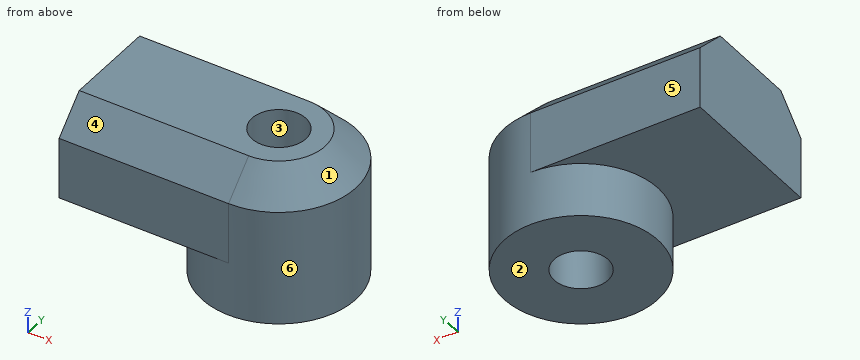
from build123d import *

# Parameters (mm, degrees)
F1_DEPTH = 6
F2_R     = 5
F2_R_2   = 1.75
F3_DEPTH = 9.5
F4_SIZE  = 2


with BuildPart() as f1:
    # F0 (on Top) → F1 (new body)
    with BuildSketch(Plane.XY):
        with BuildLine():
            ThreePointArc((0, -5), (-5, 0), (0, 5))
            Line((0, 5), (-11, 5))
            Line((-11, 5), (-11, -5))
            Line((-11, -5), (0, -5))
        make_face()
    extrude(amount=-F1_DEPTH)

    # F2 (on Top) → F3 (join)
    with BuildSketch(Plane.XY):
        Circle(F2_R)
        Circle(F2_R_2, mode=Mode.SUBTRACT)
    extrude(amount=-F3_DEPTH)

    # F4
    f4_edges = [f1.edges().sort_by_distance(p)[0] for p in [
        (-5.5, 5, 0),
    ]]
    chamfer(f4_edges, length=F4_SIZE)


solid = f1.part
Design review of the part built by this model. Coordinates are the model's own, in mm. Face numbers are marked on the shaded views. A direction names the side the tool comes from. Round coordinates to 2 decimals unless told otherwise and drop trailing zeros. Write each loop counter-clockwise with the first axis right and the second up, starting at its lowest first coordinate (ties: lowest second). Pieces come first, ordered by that corner, then holes. Notation, with made-up numbers: M -0.5,-36.75 L 47.5,-36.75 A32 ccw 47.5,-7.75 Z; hole C -34,-10 d10. An arc over 180 degrees is marked long. One line per item, written item: value. Start each with the question number.
1. Clearance check with flat-ended pins moving along their axes: P1, Ø1.5, axis at y = -1.5, z = -8, coming from the +X side; P2, Ø2, axis at y = -3, z = -7.5, coming from the +X side. State where each tip first meets the part, or that it passes through.
2. Draft analysis for pull direction Y (two halves, no side actions). For the marked faces 1, 2, 3 and 4, state which applies: pulls with the +Y half, pulls with the -Y half, needs draft (parallel to the pull), parting line crosses it, or undercut.
3. Take a section at D-D on z = -5. State the section outline as (x, y) points, then the cut area to 3 significant figures.
4. To check wall thickness, follow probe 1 along Z at (x, y) = (-9.5, -0.5); probe 2 along X at (y, z) = (0.25, -5.5); probe 3 along X at (y, z) = (-1.5, -6.75). State the ranges of each line that lie inside material, in increasing order. Write a range as from..to.
5. For the marked faces 5 and 6, list the 3-axis set-ups (+Z, -Z, +X, -X, +Y, -Y) from which the entire face can be reached by the end or side of a thin tool; tool diameter is ignored.
6. Take a section at C-C on x = -6.75. State the section outline as (y, z) points.
7. Take a section at A-A on y = 0. State the section outline as (x, z) points, then the cut area to 4 significant figures.
8. Take a section at B-B on z = -0.5. State the section outline as (x, y) points.
Computed:
1. P1: stops at x = 4.94
1. P2: stops at x = 4.58
2. face 1: parting line crosses it
2. face 2: needs draft
2. face 3: undercut
2. face 4: pulls with the -Y half
3. outline: M -11,-5 L 0,-5 A5 ccw 0,5 L -11,5 Z; hole C 0,0 d3.5
3. area: 140 mm²
4. probe 1: z = -6..0
4. probe 2: x = -11..-1.73, 1.73..4.99
4. probe 3: x = -4.77..-0.9, 0.9..4.77
5. face 5: +Z, -Z, +X, -X, +Y
5. face 6: -Z
6. outline: M -5,-6 L 5,-6 L 5,-2 L 3,0 L -3,0 L -5,-2 Z
7. outline: M -11,-6 L -5,-6 L -5,-9.5 L -1.75,-9.5 L -1.75,0 L -11,0 Z; M 1.75,-9.5 L 5,-9.5 L 5,-2 L 3,0 L 1.75,0 Z
7. area: 95.75 mm²
8. outline: M -11,-3.5 L 0,-3.5 A3.5 ccw 0,3.5 L -11,3.5 Z; hole C 0,0 d3.5
